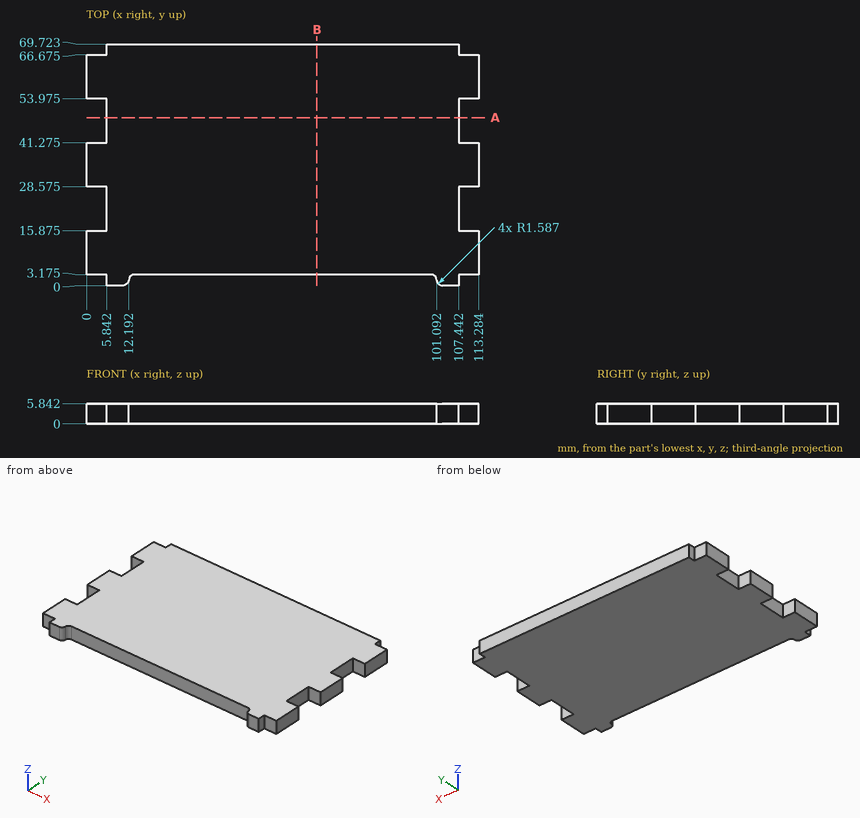
Drawing for the job (mm, zero at the part's lowest x, y, z). Coordinates: 2 decimals unless noted, no trailing zeros. Loops run counter-clockwise (first coordinate to the right, second up) from the corner with the lowest first, then second, coordinate; pieces in that order, holes last. Notation, with made-up numbers: (-22.75, -17) - (27.25, -17) arc R17 cw to (27.25, -1) - close; hole circle Ø9 at (80, 2.5). An arc over 180 degrees is marked (long way). Use CSV: the item, a comma, the result in double quotes. Start each with the question number.
Q1. Drop flat-ended pins along their axis: P1, Ø1.6, axis at y = 2, z = 2, coming from the -X side; P2, Ø0.9, axis at y = 68, z = 3.5, coming from the +X side; P3, Ø3, axis at x = 3.5, z = 4, coming from the -Y side (1 decimal). Give the stop position or say it passes through.
Q2. Cut at B-B, the plane x = 66.5. List the corners of the cut face in (y, z) (1 decimal).
Q3. Cut at A-A, the plane y = 48.5. List the corners of the cut face in (x, z).
Q4. Probe probe 1 along Y at (x, z) = (34, 0.7) (1 decimal); probe 2 along X at (y, z) = (49.5, 1.25); probe 3 along Y at (x, z) = (11, 2.35). List the from-to ranges inside material, lowest first. Write a range as from..to.
Here are the results:
1,P1,"x = 5.84"
1,P2,"x = 107.44"
1,P3,"y = 3.2"
2,outline,"(3.2, 0) - (69.7, 0) - (69.7, 5.8) - (3.2, 5.8) - close"
3,outline,"(5.84, 0) - (107.44, 0) - (107.44, 5.84) - (5.84, 5.84) - close"
4,probe 1,"3.2..69.7"
4,probe 2,"5.84..107.44"
4,probe 3,"0.05..69.72"
